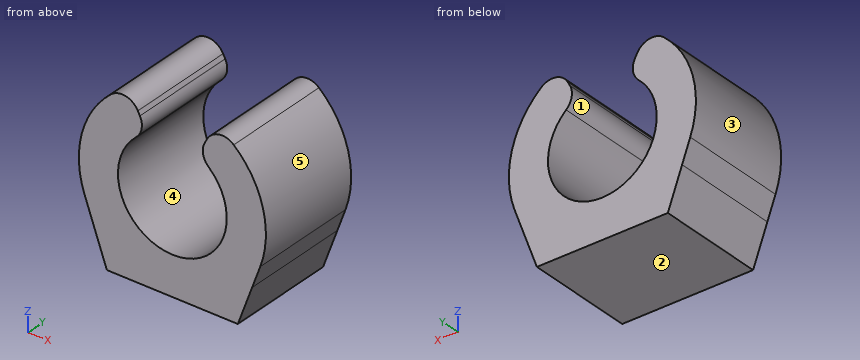
```python
from build123d import *

# Parameters (mm, degrees)
F1_DEPTH = 2.5


with BuildPart() as f1:
    # F0 (on Front) → F1 (new body, symmetric)
    with BuildSketch(Plane.XZ):
        with BuildLine():
            ThreePointArc((0, -2.5), (-2.3354308974, -0.8920552244), (-1.6666666667, 1.8633899812))
            ThreePointArc((-1.6666666667, 1.8633899812), (-1.4126546867, 2.3179448999), (-1.49220925, 2.8325450666))
            Line((-1.49220925, 2.8325450666), (-1.5881221571, 3.0146090981))
            ThreePointArc((-1.5881221571, 3.0146090981), (-2.1485753305, 3.4280540352), (-2.8206930002, 3.2455648197))
            ThreePointArc((-2.8206930002, 3.2455648197), (-4.1629749971, 1.0768654389), (-4.0406782694, -1.4706866163))
            ThreePointArc((-4.0406782694, -1.4706866163), (-3.8045948422, -2.0037609855), (-3.4985711369, -2.5))
            Line((-3.4985711369, -2.5), (0, -2.5))
        make_face()
        with BuildLine():
            ThreePointArc((1.6666666667, 1.8633899812), (2.3354308974, -0.8920552244), (0, -2.5))
            Line((0, -2.5), (3.4985711369, -2.5))
            ThreePointArc((3.4985711369, -2.5), (3.8045948422, -2.0037609855), (4.0406782694, -1.4706866163))
            ThreePointArc((4.0406782694, -1.4706866163), (4.1629749971, 1.0768654389), (2.8206930002, 3.2455648197))
            ThreePointArc((2.8206930002, 3.2455648197), (2.1485753305, 3.4280540352), (1.5881221571, 3.0146090981))
            Line((1.5881221571, 3.0146090981), (1.49220925, 2.8325450666))
            ThreePointArc((1.49220925, 2.8325450666), (1.4126546867, 2.3179448999), (1.6666666667, 1.8633899812))
        make_face()
        with BuildLine():
            Line((-3.666038836, -2.5), (-3.4985711369, -2.5))
            ThreePointArc((-3.4985711369, -2.5), (-3.8045948422, -2.0037609855), (-4.0406782694, -1.4706866163))
            Line((-4.0406782694, -1.4706866163), (-3.666038836, -2.5))
        make_face()
        with BuildLine():
            ThreePointArc((0, -4.3), (-1.9672315573, -3.8236108589), (-3.4985711369, -2.5))
            Line((-3.4985711369, -2.5), (-3.666038836, -2.5))
            Line((-3.666038836, -2.5), (-3.0108924143, -4.3))
            Line((-3.0108924143, -4.3), (0, -4.3))
        make_face()
        with BuildLine():
            Line((3.666038836, -2.5), (3.4985711369, -2.5))
            ThreePointArc((3.4985711369, -2.5), (1.9672315573, -3.8236108589), (0, -4.3))
            Line((0, -4.3), (3.0108924143, -4.3))
            Line((3.0108924143, -4.3), (3.666038836, -2.5))
        make_face()
        with BuildLine():
            Line((3.4985711369, -2.5), (0, -2.5))
            Line((0, -2.5), (-3.4985711369, -2.5))
            ThreePointArc((-3.4985711369, -2.5), (-1.9672315573, -3.8236108589), (0, -4.3))
            ThreePointArc((0, -4.3), (1.9672315573, -3.8236108589), (3.4985711369, -2.5))
        make_face()
        with BuildLine():
            ThreePointArc((0, -4.3), (-1.9672315573, -3.8236108589), (-3.4985711369, -2.5))
            Line((-3.4985711369, -2.5), (-3.666038836, -2.5))
            Line((-3.666038836, -2.5), (-3.0108924143, -4.3))
            Line((-3.0108924143, -4.3), (0, -4.3))
        make_face()
        with BuildLine():
            ThreePointArc((4.0406782694, -1.4706866163), (3.8045948422, -2.0037609855), (3.4985711369, -2.5))
            Line((3.4985711369, -2.5), (3.666038836, -2.5))
            Line((3.666038836, -2.5), (4.0406782694, -1.4706866163))
        make_face()
    extrude(amount=F1_DEPTH, both=True)


solid = f1.part
```
The model under review builds one solid part; all positions refer to its coordinate system, in mm. Face numbers are marked on the shaded views. A direction names the side the tool comes from. Round coordinates to 2 decimals unless told otherwise and drop trailing zeros. Order: outer loops, then holes, each group sorted by start corner. A loop starts at its lowest first (then second) coordinate and runs counter-clockwise, first axis right, second up. Notation, with made-up numbers: (46.5, 67.25) - (88.5, 67.25) arc R32 ccw to (88.5, 105.25) - close; hole circle Ø6 at (57, 76.25). An arc over 180 degrees is marked (long way). Answer in a Markdown table with one row per item.
(1) For line 1 (X direction, y = 1.2, z = 0); line 2 (X direction, y = 0.7, z = -0.75); line 3 (Z direction, x = -2, y = 0.9) (3 decimals), list the stretches that pass through material, from the lowest coordinate up. Write a range as from..to.
Result set:
| item | result |
|---|---|
| line 1 | x = -4.3..-2.5, 2.5..4.3 |
| line 2 | x = -4.23..-2.38, 2.38..4.23 |
| line 3 | z = -4.3..-1.5, 1.5..3.385 |
(2) Take a section at C-C on x = 0. Write out the cut boundary in (y, z), plus the area to 3 significant figures.
Result set:
| item | result |
|---|---|
| outline | (-2.5, -4.3) - (2.5, -4.3) - (2.5, -2.5) - (-2.5, -2.5) - close |
| area | 9.00 mm2 |
(3) Take a section at B-B on y = 2.1. Write out the cut boundary in (x, z), plus the area to 3 significant figures.
Result set:
| item | result |
|---|---|
| outline | (-4.04, -1.47) - (-3.01, -4.3) - (3.01, -4.3) - (4.04, -1.47) arc R4.3 ccw to (2.82, 3.25) arc R0.8 ccw to (1.59, 3.01) - (1.49, 2.83) arc R0.8 ccw to (1.67, 1.86) arc R2.5 cw (long way) to (-1.67, 1.86) arc R0.8 ccw to (-1.49, 2.83) - (-1.59, 3.01) arc R0.8 ccw to (-2.82, 3.25) arc R4.3 ccw to start |
| area | 35.3 mm2 |
(4) Mouldability with a two-part tool opening along X and no side actions: class the marked faces 3, 4 and 5 as released by +X, released by -X, zero draft, split by the parting line, or undercut.
Result set:
| item | result |
|---|---|
| face 3 | released by -X |
| face 4 | undercut |
| face 5 | released by +X |
(5) Machinability: for the marked faces 1 and 2, which of the approach directions +Z, -Z, +X, -X, +Y, -Y give a long, thin tool a straight path to every point of the face, cutting with its end or side? Answer none if there is none.
Result set:
| item | result |
|---|---|
| face 1 | +Y, -Y |
| face 2 | -Z, +X, -X, +Y, -Y |
(6) Take a section at A-A on z = 0. Write out the cut boundary in (x, y), plus the area to 3 significant figures.
Result set:
| item | result |
|---|---|
| outline | (-4.3, -2.5) - (-2.5, -2.5) - (-2.5, 2.5) - (-4.3, 2.5) - close; (2.5, -2.5) - (4.3, -2.5) - (4.3, 2.5) - (2.5, 2.5) - close |
| area | 18.0 mm2 |
(7) Clearance check with flat-ended pins moving along their axes: P1, Ø2, axis at y = 0.5, z = -2.5, coming from the +X side; P2, Ø4.5, axis at x = 0, z = 0, coming from the -Y side. State where each tip first meets the part, or that it passes through.
Result set:
| item | result |
|---|---|
| P1 | stops at x = 4.03 |
| P2 | passes through |
(8) Take a section at D-D on z = 2. Write out the cut boundary in (x, y).
Result set:
| item | result |
|---|---|
| outline | (-3.81, -2.5) - (-1.55, -2.5) - (-1.55, 2.5) - (-3.81, 2.5) - close; (1.55, -2.5) - (3.81, -2.5) - (3.81, 2.5) - (1.55, 2.5) - close |
